Input: part model. Units: mm. Frame: model coordinates. A direction names the side the tool comes from. Round coordinates to 2 decimals unless told otherwise and drop trailing zeros. Write each loop counter-clockwise with the first axis right and the second up, starting at its lowest first coordinate (ties: lowest second). Pieces come first, ordered by that corner, then holes. Notation, with made-up numbers: (-30, 16.25) -> (8, 16.25) arc R17 ccw to (8, 41.25) -> close; hole circle Ø5 at (49.5, 41.25). An arc over 180 degrees is marked (long way). Write item = value, one per line.
```python
from build123d import *

# Parameters (mm, degrees)
SKETCH1_W           = 40
SKETCH1_H           = 40
BOSS_EXTRUDE1_DEPTH = 40
SKETCH2_W           = 20
SKETCH2_H           = 20
CUT_EXTRUDE1_DEPTH  = 40
CUT_EXTRUDE2_DEPTH  = 40
CUT_EXTRUDE3_DEPTH  = 40


with BuildPart() as part:
    # Sketch1 → Boss-Extrude1 (new body)
    with BuildSketch(Plane.XY):
        with Locations((20, 20)):
            Rectangle(SKETCH1_W, SKETCH1_H)
    extrude(amount=BOSS_EXTRUDE1_DEPTH)

    # Sketch2 → Cut-Extrude1 (cut)
    with BuildSketch(Plane.XY.offset(40)):
        with Locations((10, 30)):
            Rectangle(SKETCH2_W, SKETCH2_H)
    extrude(amount=-CUT_EXTRUDE1_DEPTH, mode=Mode.SUBTRACT)

    # Sketch3 → Cut-Extrude2 (cut)
    with BuildSketch(Plane.ZY.offset(-20)):
        Polygon((0, 40), (40, 20), (40, 40), align=None)
    extrude(amount=-CUT_EXTRUDE2_DEPTH, mode=Mode.SUBTRACT)

    # Sketch4 → Cut-Extrude3 (cut)
    with BuildSketch(Plane.ZY):
        Polygon((40, 20), (20, 0), (40, 0), align=None)
    extrude(amount=-CUT_EXTRUDE3_DEPTH, mode=Mode.SUBTRACT)


solid = part.part
```
1) Line query: L1, parallel to X at y = 28.5, z = 10; L2, parallel to Y at x = 7.5, z = 15; L3, parallel to Y at x = 33.5, z = 13. Output: solid intervals per line, ascending. Write a range as from..to.
Solutions:
L1 = 20..40
L2 = 0..20
L3 = 0..33.5
2) Cut plane B-B (y = 8). Return the cut outline in (x, z), and give its area (3 significant figures).
Solutions:
outline = (0, 0) -> (40, 0) -> (40, 28) -> (0, 28) -> close
area = 1,120 mm^2
3) Cut plane A-A (z = 17.5). Return the cut outline in (x, y), and give its area (4 significant figures).
Solutions:
outline = (0, 0) -> (40, 0) -> (40, 31.25) -> (20, 31.25) -> (20, 20) -> (0, 20) -> close
area = 1,025 mm^2
4) Cut plane D-D (z = 9). Return the cut outline in (x, y).
Solutions:
outline = (0, 0) -> (40, 0) -> (40, 35.5) -> (20, 35.5) -> (20, 20) -> (0, 20) -> close
5) Cut plane C-C (x = 13.5). Return the cut outline in (y, z), and give its area (3 significant figures).
Solutions:
outline = (0, 0) -> (20, 0) -> (20, 40) -> (0, 20) -> close
area = 600 mm^2
6) Access query for faces 1 (the face through (20, 10, 30)), 2 (the face through (10, 20, 20)). Directions: +Z, -Z, +X, -X, +Y, -Y. A direction counts if a zero-diameter tool reaches every point of the face in a straight line with its end or side. Return the directions, or none.
Solutions:
face_1 = +Z, +X, -X, -Y
face_2 = +Z, -Z, -X, +Y
7) First-contact query: P1, Ø6, axis at y = 27.5, z = 16.5, coming from the -X side; P2, Ø5, axis at x = 20.5, z = 28, coming from the +Y side; P3, Ø2, axis at x = 17, z = 27.5, coming from the +Y side. Flat tips, straight axial feed; report the tip coordinate or a pass-through.
Solutions:
P1 = 20
P2 = 27.25
P3 = 20
